```python
from build123d import *

# Parameters (mm, degrees)
F1_DEPTH = 63.5
F2_DEPTH = 7.9375
F0_W     = 25.4
F0_H     = 19.05
F3_DEPTH = 25.4
F5_R     = 6.35
F6_R     = 8.255
F7_DEPTH = 50.8


with BuildPart() as f1:
    # F0 (on Front) → F1 (new body, symmetric)
    with BuildSketch(Plane.XZ):
        Polygon((41.275, -9.525), (41.275, 9.525), (22.225, 9.525), (-41.275, 9.525), (-41.275, -9.525), align=None)
    extrude(amount=F1_DEPTH, both=True)

    # F0 (on Front) → F2 (join, symmetric)
    with BuildSketch(Plane.XZ):
        with BuildLine():
            Line((-41.275, 9.525), (22.225, 9.525))
            Line((22.225, 9.525), (22.225, 27.0002))
            ThreePointArc((22.225, 27.0002), (32.085462505, 51.3214784443), (56.0989919922, 61.9093822758))
            add(Edge.make_bspline(
                [(-41.275, 9.525), (-41.1447664314, 39.122666143), (14.0637717718, 61.1012042417), (56.0989919922, 61.9093822758)],
                knots=[0, 0, 0, 0, 110.5804655627, 110.5804655627, 110.5804655627, 110.5804655627], degree=3))
        make_face()
    extrude(amount=F2_DEPTH, both=True)

    # F0 (on Front) → F3 (join, symmetric)
    with BuildSketch(Plane.XZ):
        with BuildLine():
            Line((22.225, 9.525), (41.275, 9.525))
            Line((41.275, 9.525), (41.275, 27.0002))
            ThreePointArc((41.275, 27.0002), (45.9246798487, 38.2255201513), (57.15, 42.8752))
            Line((57.15, 42.8752), (60.325, 42.8752))
            Line((60.325, 42.8752), (60.325, 61.9252))
            Line((60.325, 61.9252), (57.15, 61.9252))
            add(Edge.make_bspline(
                [(56.0989919922, 61.9093822758), (56.450261188, 61.9161358517), (56.8006104667, 61.9214110624), (57.15, 61.9252)],
                knots=[110.5804655627, 110.5804655627, 110.5804655627, 110.5804655627, 111.5045361635, 111.5045361635, 111.5045361635, 111.5045361635], degree=3))
            ThreePointArc((56.0989919922, 61.9093822758), (32.085462505, 51.3214784443), (22.225, 27.0002))
            Line((22.225, 27.0002), (22.225, 9.525))
        make_face()
        with Locations((73.025, 52.4002)):
            Rectangle(F0_W, F0_H)
    extrude(amount=F3_DEPTH, both=True)

    # F0 (on Front) → F4 (revolve)
    with BuildSketch(Plane.XZ):
        Polygon((85.725, 61.9252), (85.725, 42.8752), (85.725, 38.1), (111.125, 38.1), (111.125, 66.675), (85.725, 66.675), align=None)
    revolve(axis=Axis((85.725, 0, 52.3875), (0, 0, 1)))

    # F5
    f5_edges = [f1.edges().sort_by_distance(p)[0] for p in [
        (-41.275, -63.5, 0),
        (41.275, -63.5, 0),
        (41.275, 63.5, 0),
        (-41.275, 63.5, 0),
    ]]
    fillet(f5_edges, radius=F5_R)

    # F6 (on face) → F7 (join)
    with BuildSketch(Plane.XY.offset(66.675)):
        with Locations((85.725, 0)):
            Circle(F6_R)
    extrude(amount=-F7_DEPTH)


solid = f1.part
```
The listing builds one solid part. Answer for the finished solid, in the listing's coordinates (mm). A direction names the side the tool comes from. Coordinates: 2 decimals unless noted, no trailing zeros. Loops run counter-clockwise (first coordinate to the right, second up) from the corner with the lowest first, then second, coordinate; pieces in that order, holes last. Notation, with made-up numbers: M 58.5,-16.5 L 103.5,-16.5 A23 ccw 103.5,19.5 Z; hole C -30.75,16 d1. An arc over 180 degrees is marked long. Answer as CSV lines item,"result". Start each with the question number.
(1) The mould has two halves that part along X. Classify faces 6 (the flat face through (1, -36, 9.525)), 7 (the flat face through (22.225, -17, 18)), 8 (the flat face through (92, 6, 38.1)): pulls with the +X half, pulls with the -X half, needs draft (parallel to the pull), parting line crosses it, or undercut.
(2) Find the intervals of material crossed by L1, parallel to Y at x = 39, z = 30; L2, parallel to Z at x = -1.5, y = -24.5 (3 decimals); L3, parallel to Y at x = 15, z = 44.5, in increasing order. Write a range as [from, to].
(3) For faces 1 (the cylindrical face through (45.8, -0.4, 38.1)), 2 (the cylindrical face through (32.35, -16.79, 51.59)), 3 (the flat face through (60, -2, 61.925)), 4 (the flat face through (1, 35, 9.525)), 5 (the flat face through (46, -25.4, 42)), determine the directions among +Z, -Z, +X, -X, +Y, -Y from which every point of the face is accessible in a straight line to the end or side of a thin tool.
(4) Given pin 1 (11 mm diameter, centred on y = 1.5, z = 12.5, fed in from +X); pin 2 (5 mm diameter, centred on x = 82, y = 2.5, fed in from -Z) (3 decimals); pin 3 (16.5 mm diameter, centred on x = 18.5, y = 22.5, fed in from +Z), each flat-ended and moving along its own axis, determine where each tip first touches the part or whether it passes through.
(5) The part is cut by section A-A (x = 74). Give the vertices of the cut face in (y, z) (3 decimals), and give its area (3 significant figures).
Determined:
1,face 6,"needs draft"
1,face 7,"pulls with the -X half"
1,face 8,"undercut"
2,L1,"[-25.4, 25.4]"
2,L2,"[-9.525, 9.525]"
2,L3,"[-7.94, 7.94]"
3,face 1,"-Z, +Y, -Y"
3,face 2,"+Z, -X, -Y"
3,face 3,"+Z, -X"
3,face 4,"+Z, -X, +Y"
3,face 5,"+Z, +X, -X, -Y"
4,pin 1,"x = 93.98"
4,pin 2,"z = 15.875"
4,pin 3,"z = 44.19"
5,outline,"M -25.4,42.875 L -22.532,42.875 L -22.532,38.1 L 22.532,38.1 L 22.532,42.875 L 25.4,42.875 L 25.4,61.925 L 22.532,61.925 L 22.532,66.675 L -22.532,66.675 L -22.532,61.925 L -25.4,61.925 Z"
5,area,"1,400 mm2"
